Verification items for the finished model (mm, model axes). Face numbers are marked on the shaded views. A direction names the side the tool comes from. Coordinates: 2 decimals unless noted, no trailing zeros. Write each loop counter-clockwise with the first axis right and the second up, starting at its lowest first coordinate (ties: lowest second). Pieces come first, ordered by that corner, then holes. Notation, with made-up numbers: M -3,-37 L 15,-37 A16 cw 15,-11 Z; hole C 82,8 d10. An arc over 180 degrees is marked long. Answer in a Markdown table with one row per item.
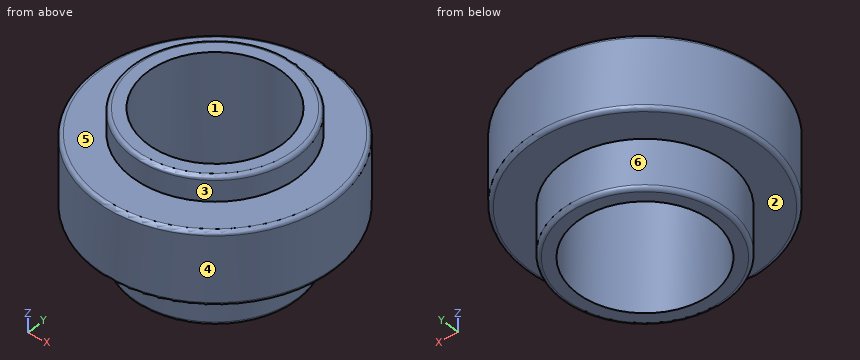
from build123d import *

# Parameters (mm, degrees)
ZAOKR_GLENIE1_R = 1


with BuildPart() as part:
    # Szkic2 → Obrót1 (revolve)
    with BuildSketch(Plane(origin=(0, 0, 0), x_dir=(0, 0, -1), z_dir=(1, 0, 0)), mode=Mode.PRIVATE) as obr_t1_sk:
        Polygon((-9.5, 21.5), (-9.5, 31), (9.5, 31), (9.5, 21.5), (22.2, 21.5), (22.2, 17.5), (-15.9, 17.5), (-15.9, 21.5), align=None)
    revolve(obr_t1_sk.sketch.rotate(Axis((0, 0, 23.470588235), (0, 0, -1)), 90), axis=Axis((0, 0, 23.470588235), (0, 0, -1)))

    # Zaokrąglenie1
    zaokr_glenie1_edges = [part.edges().sort_by_distance(p)[0] for p in [
        (-21.5, 0, 15.9),
        (-31, 0, 9.5),
        (-31, 0, -9.5),
        (-21.5, 0, -22.2),
    ]]
    fillet(zaokr_glenie1_edges, radius=ZAOKR_GLENIE1_R)


solid = part.part
1) Release check for a two-part mould opening along Y. For the marked faces 1, 2 and 3 record: +Y half, -Y half, draft (parallel to the pull), parting line (faces both ways), or undercut.
Response values:
| item | result |
|---|---|
| face 1 | undercut |
| face 2 | draft |
| face 3 | parting line |
2) Tool access check on the marked faces 4, 5 and 6. Record the directions out of +Z, -Z, +X, -X, +Y, -Y that give a thin tool (end or side, any length) a straight path to the whole face; none if there is none.
Response values:
| item | result |
|---|---|
| face 4 | +Z, -Z |
| face 5 | +Z |
| face 6 | -Z |
3) Depth check by flat-ended pin: pin 1 (4 mm diameter, centred on x = 15.5, z = 2, fed in from -Y); pin 2 (6 mm diameter, centred on y = 17, z = -16.5, fed in from +X); pin 3 (4 mm diameter, centred on y = -10.5, z = -16, fed in from +X); pin 4 (5 mm diameter, centred on x = -19, y = -10.5, fed in from +Z). Enter the tip coordinate at first touch or a pass-through.
Response values:
| item | result |
|---|---|
| pin 1 | stops at y = -27.91 |
| pin 2 | stops at x = 16.32 |
| pin 3 | stops at x = 19.75 |
| pin 4 | stops at z = 15.9 |
4) Sectioned sample at A-A (y = 0). Record the cut outline in (x, z).
Response values:
| item | result |
|---|---|
| outline | M -31,-8.5 A1 ccw -30,-9.5 L -21.5,-9.5 L -21.5,-21.2 A1 ccw -20.5,-22.2 L -17.5,-22.2 L -17.5,15.9 L -20.5,15.9 A1 ccw -21.5,14.9 L -21.5,9.5 L -30,9.5 A1 ccw -31,8.5 Z; M 17.5,-22.2 L 20.5,-22.2 A1 ccw 21.5,-21.2 L 21.5,-9.5 L 30,-9.5 A1 ccw 31,-8.5 L 31,8.5 A1 ccw 30,9.5 L 21.5,9.5 L 21.5,14.9 A1 ccw 20.5,15.9 L 17.5,15.9 Z |
5) Sectioned sample at D-D (z = -12). Record the cut outline in (x, y).
Response values:
| item | result |
|---|---|
| outline | C 0,0 d43; hole C 0,0 d35 |
6) Sectioned sample at C-C (z = -2). Record the cut outline in (x, y).
Response values:
| item | result |
|---|---|
| outline | C 0,0 d62; hole C 0,0 d35 |
7) Thickness scan on L1, parallel to Y at x = 0, z = 7; L2, parallel to Z at x = -9, y = -24.5; L3, parallel to X at y = -13.5, z = 9. Record the ranges inside material, lowest first. Write a range as [from, to].
Response values:
| item | result |
|---|---|
| L1 | y = [-31, -17.5], [17.5, 31] |
| L2 | z = [-9.5, 9.5] |
| L3 | x = [-27.76, -11.14], [11.14, 27.76] |
